Design review of the part built by this model. Coordinates are the model's own, in mm. Face numbers are marked on the shaded views. A direction names the side the tool comes from. Coordinates: 2 decimals unless noted, no trailing zeros. Loops run counter-clockwise (first coordinate to the right, second up) from the corner with the lowest first, then second, coordinate; pieces in that order, holes last. Notation, with made-up numbers: (46.25, -8) -> (80.25, -8) arc R29 ccw to (80.25, 25) -> close; hole circle Ø9 at (8, -24). An arc over 180 degrees is marked (long way). Use a Markdown table: item, result. Add a question column.
Q1. Clearance check with flat-ended pins moving along their axes: pin 1 Ø2 at (x, z) = (-66.5, 56.5) entering from -Y (3 decimals); pin 2 Ø8 at (x, y) = (-119.5, -7.5) entering from -Z (3 decimals). State where each tip first meets the part, or that it passes through.
Q2. For probe 1 along X at (y, z) = (-29, 29) (3 decimals); probe 2 along Z at (x, y) = (-54.5, -2); probe 3 along X at (y, z) = (-3, -37), list the stretches that pass through material, from the lowest coordinate up.
Q3. Take a section at C-C on y = -29.5. Write out the cut boundary in (x, z) (3 decimals).
Q4. For the marked faces 5 and 6, list the 3-axis set-ups (+Z, -Z, +X, -X, +Y, -Y) from which the entire face can be reached by the end or side of a thin tool; tool diameter is ignored.
Q5. Draft analysis for pull direction X (two halves, no side actions). For the marked faces 1, 2, 3 and 4, state which applies: pulls with the +X half, pulls with the -X half, needs draft (parallel to the pull), parting line crosses it, or undercut.
Q6. Take a section at A-A on x = -122.5. Write out the cut boundary in (y, z) (3 decimals), plus the area to 3 significant figures.
Q7. Take a section at B-B on z = -32. Write out the cut boundary in (x, y) (3 decimals), plus the area to 3 significant figures.
Q8. Take a section at D-D on z = -61.5. Write out the cut boundary in (x, y) (3 decimals).
from build123d import *

# Parameters (mm, degrees)
F0_W     = 381
F0_H     = 152.4
F1_DEPTH = 38.1
F2_T     = -3.175
F3_W     = 304.8
F3_H     = 95.25
F4_DEPTH = 25.4


with BuildPart() as f1:
    # F0 (on Front) → F1 (new body)
    with BuildSketch(Plane.XZ):
        Rectangle(F0_W, F0_H)
    extrude(amount=F1_DEPTH)

    # F2
    f2_openings = [f1.faces().sort_by_distance(p)[0] for p in [
        (0, -38.1, 0),
        (0, -19.05, -76.2),
    ]]
    offset(amount=F2_T, openings=f2_openings)

    # F3 (on face) → F4 (cut)
    with BuildSketch(Plane.XZ.offset(3.175)):
        with Locations((0, -9.525)):
            Rectangle(F3_W, F3_H)
    extrude(amount=-F4_DEPTH, mode=Mode.SUBTRACT)


solid = f1.part
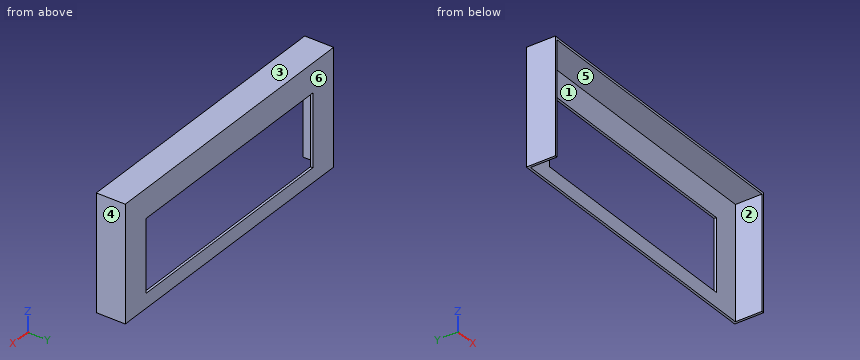
Answer list:
| question | item | result |
|---|---|---|
| 1 | pin 1 | y = -3.175 |
| 1 | pin 2 | z = 73.025 |
| 2 | probe 1 | -190.5 to -187.325, 187.325 to 190.5 |
| 2 | probe 2 | -76.2 to -57.15, 38.1 to 76.2 |
| 2 | probe 3 | -190.5 to -152.4, 152.4 to 190.5 |
| 3 | outline | (-190.5, -76.2) -> (-187.325, -76.2) -> (-187.325, 73.025) -> (187.325, 73.025) -> (187.325, -76.2) -> (190.5, -76.2) -> (190.5, 76.2) -> (-190.5, 76.2) -> close |
| 4 | face 5 | -Z, -Y |
| 4 | face 6 | +Z, -Z, +X, -X, +Y |
| 5 | face 1 | undercut |
| 5 | face 2 | undercut |
| 5 | face 3 | needs draft |
| 5 | face 4 | pulls with the +X half |
| 6 | outline | (-38.1, 73.025) -> (-3.175, 73.025) -> (-3.175, 38.1) -> (0, 38.1) -> (0, 76.2) -> (-38.1, 76.2) -> close; (-3.175, -76.2) -> (0, -76.2) -> (0, -57.15) -> (-3.175, -57.15) -> close |
| 6 | area | 292 mm² |
| 7 | outline | (-190.5, -38.1) -> (-187.325, -38.1) -> (-187.325, -3.175) -> (-152.4, -3.175) -> (-152.4, 0) -> (-190.5, 0) -> close; (152.4, -3.175) -> (187.325, -3.175) -> (187.325, -38.1) -> (190.5, -38.1) -> (190.5, 0) -> (152.4, 0) -> close |
| 7 | area | 464 mm² |
| 8 | outline | (-190.5, -38.1) -> (-187.325, -38.1) -> (-187.325, -3.175) -> (187.325, -3.175) -> (187.325, -38.1) -> (190.5, -38.1) -> (190.5, 0) -> (-190.5, 0) -> close |
